from build123d import *

# Parameters (mm, degrees)
SKETCH2_W                        = 60
SKETCH2_H                        = 60
BOSS_EXTRUDE1_DEPTH              = 10
SKETCH7_W                        = 28.32
SKETCH7_H                        = 16.5
CUT_EXTRUDE2_DEPTH               = 44.588989435
FILLET2_R                        = 2
CBORE_FOR_M2_5_SHCS2_D           = 3.1
CBORE_FOR_M2_5_SHCS2_CBORE_D     = 5.5
CBORE_FOR_M2_5_SHCS2_CBORE_DEPTH = 2.5
MOVE_FACE1_BY                    = 3.5
MOVE_FACE1_2_BY                  = 3.5
MOVE_FACE1_3_BY                  = 3.5
MOVE_FACE1_4_BY                  = 3.5
SKETCH11_W                       = 10
SKETCH11_H                       = 24.3
BOSS_EXTRUDE2_DEPTH              = 60
SKETCH12_W                       = 20
SKETCH12_H                       = 60
BOSS_EXTRUDE3_DEPTH              = 10
CBORE_FOR_M4_SHCS1_D             = 4.8
CBORE_FOR_M4_SHCS1_CBORE_D       = 8
CBORE_FOR_M4_SHCS1_CBORE_DEPTH   = 4
FILLET5_R                        = 2


with BuildPart() as part:
    # Sketch2 → Boss-Extrude1 (new body)
    with BuildSketch(Plane(origin=(0, 0, 0), x_dir=(1, 0, 0), z_dir=(0, 1, 0))):
        Rectangle(SKETCH2_W, SKETCH2_H)
    extrude(amount=BOSS_EXTRUDE1_DEPTH)

    # Sketch7 → Cut-Extrude2 (cut, through all)
    with BuildSketch(Plane(origin=(0, 10, 0), x_dir=(1, 0, 0), z_dir=(0, 1, 0))):
        Rectangle(SKETCH7_W, SKETCH7_H)
    extrude(amount=-CUT_EXTRUDE2_DEPTH, mode=Mode.SUBTRACT)

    # Fillet2
    fillet2_edges = [part.edges().sort_by_distance(p)[0] for p in [
        (-14.16, 5, 8.25),
        (-14.16, 5, -8.25),
        (14.16, 5, -8.25),
        (14.16, 5, 8.25),
    ]]
    fillet(fillet2_edges, radius=FILLET2_R)

    # CBORE for M2.5 SHCS2 (through all)
    with Locations(Plane(origin=(0, 0, 0), x_dir=(-1, 0, 0), z_dir=(0, -1, 0))):
        with Locations((11, -20), (-11, -20), (11, 20), (-11, 20)):
            CounterBoreHole(CBORE_FOR_M2_5_SHCS2_D / 2, CBORE_FOR_M2_5_SHCS2_CBORE_D / 2, CBORE_FOR_M2_5_SHCS2_CBORE_DEPTH)

    # Move Face1: a face moved inward by 3.5
    extrude(part.faces().sort_by_distance((11, 2.5, 22.2))[0], amount=MOVE_FACE1_BY, dir=(0, 1, 0), mode=Mode.SUBTRACT)

    # Move Face1 2: a face moved inward by 3.5
    extrude(part.faces().sort_by_distance((-11, 2.5, 22.2))[0], amount=MOVE_FACE1_2_BY, dir=(0, 1, 0), mode=Mode.SUBTRACT)

    # Move Face1 3: a face moved inward by 3.5
    extrude(part.faces().sort_by_distance((11, 2.5, -17.8))[0], amount=MOVE_FACE1_3_BY, dir=(0, 1, 0), mode=Mode.SUBTRACT)

    # Move Face1 4: a face moved inward by 3.5
    extrude(part.faces().sort_by_distance((-11, 2.5, -17.8))[0], amount=MOVE_FACE1_4_BY, dir=(0, 1, 0), mode=Mode.SUBTRACT)

    # Sketch11 → Boss-Extrude2 (add)
    with BuildSketch(Plane(origin=(0, 0, -30), x_dir=(-1, 0, 0), z_dir=(0, 0, -1))):
        with Locations((-25, -12.15)):
            Rectangle(SKETCH11_W, SKETCH11_H)
    boss_extrude2 = extrude(amount=-BOSS_EXTRUDE2_DEPTH)

    # Sketch12 → Boss-Extrude3 (add)
    with BuildSketch(Plane.XZ.offset(24.3)):
        with Locations((40, 0)):
            Rectangle(SKETCH12_W, SKETCH12_H)
    boss_extrude3 = extrude(amount=-BOSS_EXTRUDE3_DEPTH)

    # CBORE for M4 SHCS1 (through all)
    with Locations(Plane(origin=(0, -14.3, 0), x_dir=(1, 0, 0), z_dir=(0, 1, 0))):
        with Locations((40, 20), (40, -20)):
            cbore_for_m4_shcs1 = CounterBoreHole(CBORE_FOR_M4_SHCS1_D / 2, CBORE_FOR_M4_SHCS1_CBORE_D / 2, CBORE_FOR_M4_SHCS1_CBORE_DEPTH)

    # Mirror1: Boss-Extrude2, Boss-Extrude3, CBORE for M4 SHCS1 across plane
    add(boss_extrude2.mirror(Plane(origin=(0, 0, 0), x_dir=(0, 0, 1), z_dir=(1, 0, 0))))
    add(boss_extrude3.mirror(Plane(origin=(0, 0, 0), x_dir=(0, 0, 1), z_dir=(1, 0, 0))))
    add(cbore_for_m4_shcs1.mirror(Plane(origin=(0, 0, 0), x_dir=(0, 0, 1), z_dir=(1, 0, 0))), mode=Mode.SUBTRACT)

    # Fillet5
    fillet5_edges = [part.edges().sort_by_distance(p)[0] for p in [
        (50, -14.3, 0),
        (30, -14.3, 0),
        (30, 10, 0),
        (-20, 0, 0),
        (-20, -24.3, 0),
        (-30, -14.3, 0),
        (-50, -14.3, 0),
        (-30, 10, 0),
        (20, 0, 0),
        (20, -24.3, 0),
    ]]
    fillet(fillet5_edges, radius=FILLET5_R)


solid = part.part
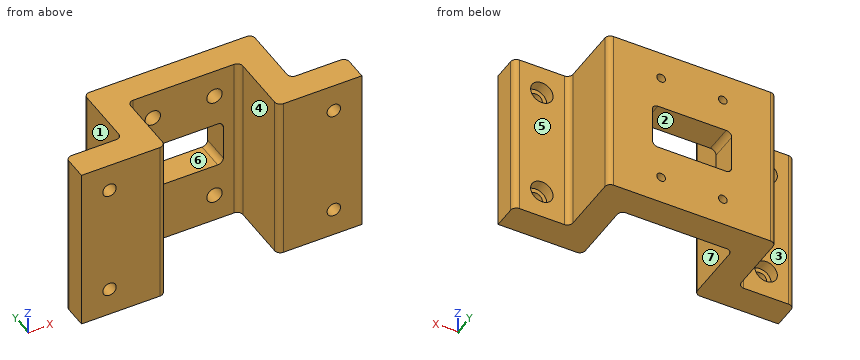
The model under review builds one solid part; all positions refer to its coordinate system, in mm. Face numbers are marked on the shaded views. A direction names the side the tool comes from. Round coordinates to 2 decimals unless told otherwise and drop trailing zeros. Order: outer loops, then holes, each group sorted by start corner. A loop starts at its lowest first (then second) coordinate and runs counter-clockwise, first axis right, second up. Notation, with made-up numbers: (22.25, -31.5) -> (47.25, -31.5) arc R26 ccw to (47.25, -17.5) -> close; hole circle Ø5 at (53, 46.25). An arc over 180 degrees is marked (long way). Write item = value, one per line. Start each with the question number.
Item 1: Clearance check with flat-ended pins moving along their axes: pin 1 Ø10 at (y, z) = (-10.5, 19.5) entering from +X; pin 2 Ø7.5 at (x, z) = (-40, 20) entering from -Y; pin 3 Ø5.5 at (x, z) = (40, -20) entering from +Y; pin 4 Ø6.5 at (x, z) = (38.5, -21.5) entering from +Y. State where each tip first meets the part, or that it passes through.
Item 2: Consider section B-B on y = -5. Write out the cut boundary in (x, z), plus the area to 3 significant figures.
Item 3: Consider section A-A on x = -11. Write out the cut boundary in (y, z).
Item 4: For line 1 along Z through (x, y) = (-11, 1.25); line 2 along Z through (x, y) = (11, 7.2); line 3 along Z through (x, y) = (-40, -20.7), list the stretches that pass through material, from the lowest coordinate up.
Item 5: Mouldability with a two-part tool opening along X and no side actions: class the marked faces 1, 2, 3 and 4 as released by +X, released by -X, zero draft, split by the parting line, or undercut.
Item 6: For the marked faces 5, 6 and 7, list the 3-axis set-ups (+Z, -Z, +X, -X, +Y, -Y) from which the entire face can be reached by the end or side of a thin tool; tool diameter is ignored.
Item 7: Consider section D-D on z = -20. Count the separate pieces of the cut face and the enclosed holes in it, plus the area to 3 significant figures.
Item 8: Consider section C-C on z = -12. Write out the cut boundary in (x, y), plus the area to 3 significant figures.
Conclusion:
q1.pin_1 = 49.83
q1.pin_2 = -24.3
q1.pin_3 = -18.3
q1.pin_4 = -14.3
q2.outline = (-30, -30) -> (-20, -30) -> (-20, 30) -> (-30, 30) -> close; (20, -30) -> (30, -30) -> (30, 30) -> (20, 30) -> close
q2.area = 1,200 mm2
q3.outline = (0, -30) -> (10, -30) -> (10, -21.55) -> (6, -21.55) -> (6, -22.75) -> (0, -22.75) -> close; (0, -17.25) -> (6, -17.25) -> (6, -18.45) -> (10, -18.45) -> (10, -8.25) -> (0, -8.25) -> close; (0, 8.25) -> (10, 8.25) -> (10, 18.45) -> (6, 18.45) -> (6, 17.25) -> (0, 17.25) -> close; (0, 22.75) -> (6, 22.75) -> (6, 21.55) -> (10, 21.55) -> (10, 30) -> (0, 30) -> close
q4.line_1 = -30 to -22.75, -17.25 to -8.25, 8.25 to 17.25, 22.75 to 30
q4.line_2 = -30 to -21.55, -18.45 to -8.25, 8.25 to 18.45, 21.55 to 30
q4.line_3 = -30 to -22.4, -17.6 to 17.6, 22.4 to 30
q5.face_1 = released by -X
q5.face_2 = undercut
q5.face_3 = zero draft
q5.face_4 = undercut
q6.face_5 = +Z, -Z, +X, +Y
q6.face_6 = +Y, -Y
q6.face_7 = +Z, -Z, -Y
q7.separate_pieces = 5
q7.enclosed_holes = 0
q7.area = 1,270 mm2
q8.outline = (-50, -24.3) -> (-22, -24.3) arc R2 ccw to (-20, -22.3) -> (-20, -2) arc R2 cw to (-18, 0) -> (18, 0) arc R2 cw to (20, -2) -> (20, -22.3) arc R2 ccw to (22, -24.3) -> (50, -24.3) -> (50, -16.3) arc R2 ccw to (48, -14.3) -> (32, -14.3) arc R2 cw to (30, -12.3) -> (30, 8) arc R2 ccw to (28, 10) -> (-28, 10) arc R2 ccw to (-30, 8) -> (-30, -12.3) arc R2 cw to (-32, -14.3) -> (-48, -14.3) arc R2 ccw to (-50, -16.3) -> close
q8.area = 1,480 mm2
